Input: part model. Units: mm. Frame: model coordinates. Face numbers are marked on the shaded views. A direction names the side the tool comes from. Round coordinates to 2 decimals unless told otherwise and drop trailing zeros. Order: outer loops, then holes, each group sorted by start corner. A loop starts at its lowest first (then second) coordinate and runs counter-clockwise, first axis right, second up. Notation, with made-up numbers: (12, 27) - (39, 27) arc R19 ccw to (39, 49) - close; hole circle Ø1 at (38.25, 63.5). An arc over 180 degrees is marked (long way). One line per item, written item: value. Start each with the question number.
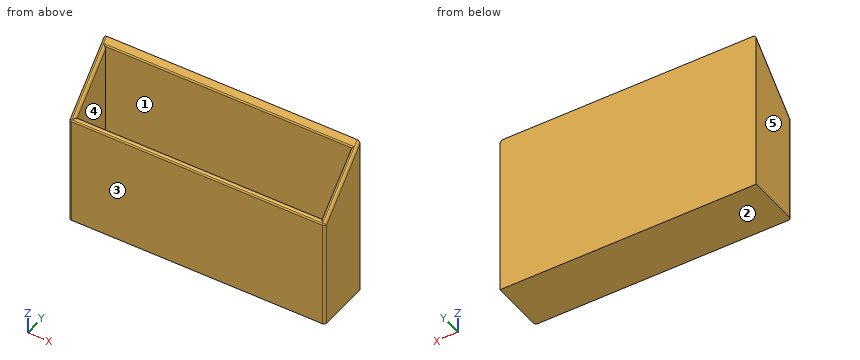
from build123d import *

# Parameters (mm, degrees)
F1_DEPTH = 59.65
F3_DEPTH = 57.15
F4_R     = 1.24999


# Not quite as in the source:
# - a fillet or chamfer is up to 0.001 mm smaller than in the source, because OpenCascade refuses the exact size


with BuildPart() as f1:
    # F0 (on Right) → F1 (new body, symmetric)
    with BuildSketch(Plane.YZ):
        Polygon((-25.4, 0), (0, 0), (0, 76.2), (-25.4, 50.8), align=None)
    extrude(amount=F1_DEPTH, both=True)

    # F2 (on Right) → F3 (cut, symmetric)
    with BuildSketch(Plane.YZ):
        Polygon((-2.5, 73.7), (-22.9, 53.3), (-22.9, 2.5), (-2.5, 2.5), align=None)
    extrude(amount=F3_DEPTH, both=True, mode=Mode.SUBTRACT)

    # F4 (radius 1.25 in the source; OpenCascade refuses exactly that, so slightly less here)
    f4_edges = [f1.edges().sort_by_distance(p)[0] for p in [
        (-59.65, -25.4, 25.4),
        (59.65, -25.4, 25.4),
        (59.65, -12.7, 63.5),
        (0, -25.4, 50.8),
        (-59.65, -12.7, 63.5),
        (57.15, -12.7, 63.5),
        (0, -22.9, 53.3),
        (0, -2.5, 73.7),
        (-57.15, -12.7, 63.5),
    ]]
    fillet(f4_edges, radius=F4_R)


solid = f1.part
Item 1: Section query A-A on z = 8. Return loops of the section in (x, y), and give its area (3 significant figures).
Item 2: First-contact query: pin 1 Ø5 at (x, z) = (42, 57) entering from -Y; pin 2 Ø5 at (x, y) = (-30.5, -10) entering from +Z. Flat tips, straight axial feed; report the tip coordinate or a pass-through.
Item 3: Line query: L1, parallel to X at y = -5.5, z = 66; L2, parallel to Y at x = -18, z = 16.5; L3, parallel to Z at x = 24, y = -9. Output: solid intervals per line, ascending.
Item 4: Pull-direction query (Y, two-part tool) for the marked faces 1, 2 and 3; classes: released by +Y, released by -Y, zero draft, split by the parting line, or undercut.
Item 5: Reachability of the marked faces 4 and 5 from +Z, -Z, +X, -X, +Y, -Y: full face, straight path, thin tool, end or side. Return the list, or none.
Geometry results:
1. outline: (-59.65, -24.15) arc R1.25 ccw to (-58.4, -25.4) - (58.4, -25.4) arc R1.25 ccw to (59.65, -24.15) - (59.65, 0) - (-59.65, 0) - close; hole (-57.15, -22.9) - (57.15, -22.9) - (57.15, -2.5) - (-57.15, -2.5) - close
1. area: 698 mm^2
2. pin 1: stops at y = -2.5
2. pin 2: stops at z = 2.5
3. L1: x = -59.65 to -57.15, 57.15 to 59.65
3. L2: y = -25.4 to -22.9, -2.5 to 0
3. L3: z = 0 to 2.5
4. face 1: undercut
4. face 2: zero draft
4. face 3: released by -Y
5. face 4: +Z
5. face 5: +Z, -Z, -X, +Y, -Y
